Can you work these out from the drawing? Everything is in mm from the part's minimum corner. A direction names the side the tool comes from. Round coordinates to 2 decimals unless told otherwise and drop trailing zeros. Loops run counter-clockwise (first coordinate to the right, second up) from the corner with the lowest first, then second, coordinate; pieces in that order, holes last. Notation, with made-up numbers: (81.25, 35) - (140.25, 35) arc R10 ccw to (140.25, 41) - close; hole circle Ø3 at (-13, 32). An arc over 180 degrees is marked (long way). Return JSON: item names as keys, results as strings. Group by question number.
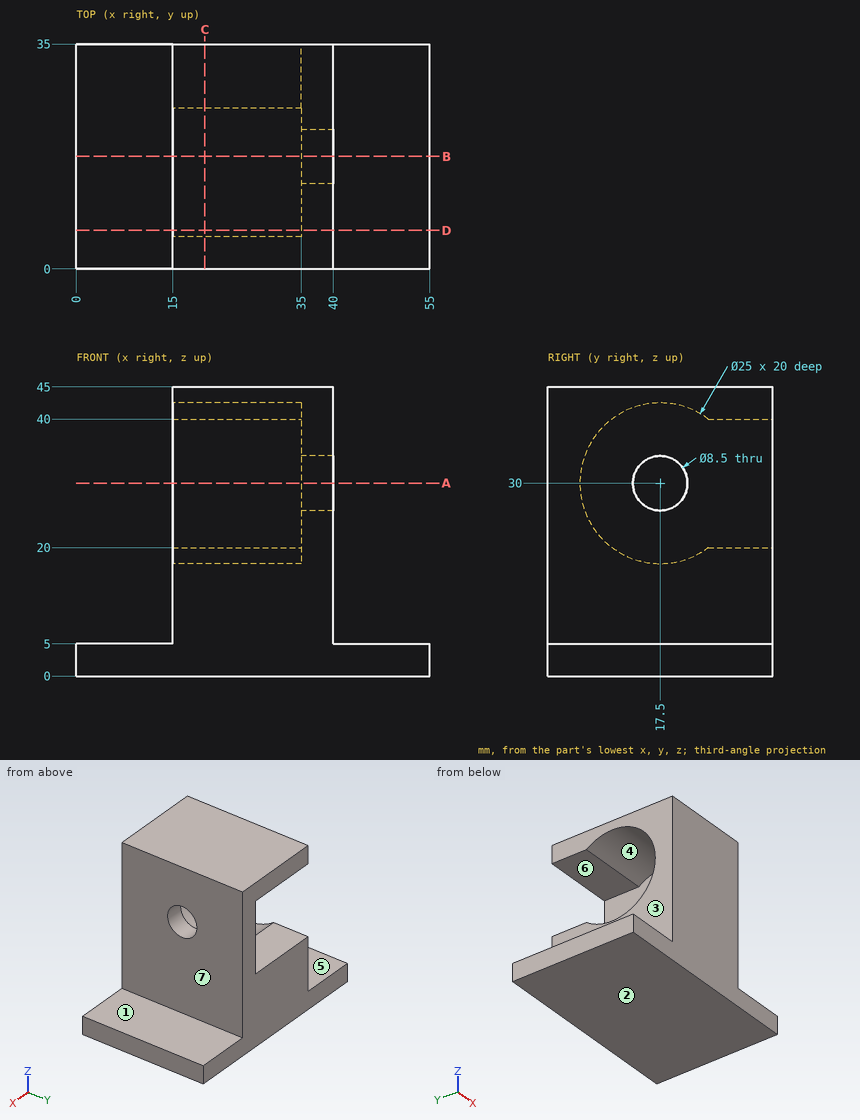
Q1. Imagine slicing it at A-A, the plane z = 30. List the corners of the cut face in (x, y) for me, and give its area (4 significant figures).
Q2. Imagine slicing it at B-B, the plane y = 17.5. List the corners of the cut face in (x, z) for me.
Q3. Will these pins go through, and if not, where does the flat tip stop? pin 1 Ø10 at (x, z) = (10.5, 18) entering from +Y; pin 2 Ø4.5 at (x, y) = (51, 10.5) entering from +Z; pin 3 Ø6 at (y, z) = (4.5, 34.5) entering from -X; pin 4 Ø10.5 at (y, z) = (19.5, 29.5) entering from +X.
Q4. Please list where these lines run through material, in increasing order: line 1 (Z direction, x = 23.25, y = 17.5); line 2 (Y direction, x = 36, z = 30); line 3 (Z direction, x = 22.5, y = 32).
Q5. Imagine slicing it at D-D, the plane y = 6. List the corners of the cut face in (x, z) for me.
Q6. For the marked faces 5, 6 and 7, which set-ups out of +Z, -Z, +X, -X, +Y, -Y let a thin tool reach every point of the face, with its end or its side?
Q7. If we mould it in two halves opening along Z, with no side actions, what happens to the marked faces 1, 2, 3 and 4? For each: +Z half, -Z half, draft (parallel to the pull), parting line (faces both ways), or undercut.
Q8. Imagine slicing it at C-C, the plane x = 20. List the corners of the cut face in (y, z) for me.
Output values:
{
 "1": {"outline": "(15, 0) - (40, 0) - (40, 13.25) - (35, 13.25) - (35, 5) - (15, 5) - close; (35, 21.75) - (40, 21.75) - (40, 35) - (35, 35) - close", "area": "232.5 mm^2"},
 "2": {"outline": "(0, 0) - (55, 0) - (55, 5) - (40, 5) - (40, 25.75) - (35, 25.75) - (35, 17.5) - (15, 17.5) - (15, 5) - (0, 5) - close; (15, 42.5) - (35, 42.5) - (35, 34.25) - (40, 34.25) - (40, 45) - (15, 45) - close"},
 "3": {"pin 1": "stops at y = 35", "pin 2": "stops at z = 5", "pin 3": "stops at x = 15", "pin 4": "stops at x = 40"},
 "4": {"line 1": "z = 0 to 17.5, 42.5 to 45", "line 2": "y = 0 to 13.25, 21.75 to 35", "line 3": "z = 0 to 20, 40 to 45"},
 "5": {"outline": "(0, 0) - (55, 0) - (55, 5) - (40, 5) - (40, 45) - (15, 45) - (15, 34.9) - (35, 34.9) - (35, 25.1) - (15, 25.1) - (15, 5) - (0, 5) - close"},
 "6": {"face 5": "+Z, -X, +Y, -Y", "face 6": "-X, +Y", "face 7": "+Z, +X, +Y, -Y"},
 "7": {"face 1": "+Z half", "face 2": "-Z half", "face 3": "draft", "face 4": "undercut"},
 "8": {"outline": "(0, 0) - (35, 0) - (35, 20) - (25, 20) arc R12.5 cw (long way) to (25, 40) - (35, 40) - (35, 45) - (0, 45) - close"}
}
